```python
from build123d import *

# Parameters (mm, degrees)
F1_DEPTH  = 6
F3_DEPTH  = 130
F5_DEPTH  = 130
F7_DEPTH  = 130
F9_DEPTH  = 6
F10_R     = 41
F11_DEPTH = 309.88


with BuildPart() as f1:
    # F0 (on Front) → F1 (new body)
    with BuildSketch(Plane.XZ):
        Polygon((-110, 0), (0, 0), (110, 0), (0, 600), align=None)
    extrude(amount=F1_DEPTH)

    # F2 (on face) → F3 (join)
    with BuildSketch(Plane(origin=(0, 0, 0), x_dir=(-1, 0, 0), z_dir=(0, 1, 0))):
        Polygon((110, 0), (106.467944, 19.265758), (0, 600), (-3.05, 583.363636), (0, 566.727273), (88.482445, 84.095757), (103.9, 0), align=None)
    extrude(amount=F3_DEPTH)

    # F4 (on face) → F5 (join)
    with BuildSketch(Plane(origin=(0, 0, 0), x_dir=(-1, 0, 0), z_dir=(0, 1, 0))):
        Polygon((0, 566.727273), (-3.05, 583.363636), (-110, 0), (-103.9, 0), (-101.40299, 13.620052), align=None)
    extrude(amount=F5_DEPTH)

    # F6 (on face) → F7 (join)
    with BuildSketch(Plane(origin=(0, 0, 0), x_dir=(-1, 0, 0), z_dir=(0, 1, 0))):
        Polygon((-102.8, 6), (-103.9, 0), (103.9, 0), (102.8, 6), (94.243981, 6), (-89.78457, 6), align=None)
    extrude(amount=F7_DEPTH)

    # F8 (on face) → F9 (join)
    with BuildSketch(Plane(origin=(0, 130, 0), x_dir=(-1, 0, 0), z_dir=(0, 1, 0))):
        Polygon((110, 0), (0, 600), (-110, 0), align=None)
    extrude(amount=F9_DEPTH)

    # F10 (on face) → F11 (cut)
    with BuildSketch(Plane.XZ.offset(6)):
        with Locations((48.797943, 51.662218)):
            Circle(F10_R)
        with Locations((-51.237836, 50.848916)):
            Circle(F10_R)
        with Locations((-0.8133, 127.299026)):
            Circle(F10_R)
        with Locations((0, 217.074677)):
            Circle(F10_R)
        with Locations((0, 306.537598)):
            Circle(F10_R)
    extrude(amount=-F11_DEPTH, mode=Mode.SUBTRACT)


solid = f1.part
```
Input: part model. Units: mm. Frame: model coordinates. A direction names the side the tool comes from. Give positions to 0.01 mm unless a question says otherwise; leave off trailing zeros. Loops run counter-clockwise (first coordinate to the right, second up) from the corner with the lowest first, then second, coordinate; pieces in that order, holes last. Notation, with made-up numbers: (-4.5, 85.25) -> (13.5, 85.25) arc R21 cw to (13.5, 103.25) -> close; hole circle Ø5 at (31.5, -2). An arc over 180 degrees is marked (long way). Use a Markdown table: item, result.
Q1. Pull-direction query (Y, two-part tool) for faces 1 (the cylindrical face through (18.919, 132.958, 270.164)), 2 (the flat face through (16, -6, 257)), 3 (the flat face through (15, 0, 267)), 4 (the flat face through (17, 136, 257)); classes: pulls with the +Y half, pulls with the -Y half, needs draft (parallel to the pull), parting line crosses it, or undercut.
Entries:
| item | result |
|---|---|
| face 1 | needs draft |
| face 2 | pulls with the -Y half |
| face 3 | undercut |
| face 4 | pulls with the +Y half |
Q2. First-contact query: P1, Ø1, axis at y = 62, z = 442.5, coming from the -X side; P2, Ø10, axis at y = 41.5, z = 71.5, coming from the +X side; P3, Ø10, axis at y = 108.5, z = 471, coming from the -X side. Flat tips, straight axial feed; report the tip coordinate or a pass-through.
Entries:
| item | result |
|---|---|
| P1 | stops at x = -28.97 |
| P2 | stops at x = 97.81 |
| P3 | stops at x = -24.57 |
Q3. Section query A-A, the plane z = 438. Return the cut outline in (x, y), plus the area to 3 significant figures.
Entries:
| item | result |
|---|---|
| outline | (-29.7, -6) -> (29.7, -6) -> (29.7, 136) -> (-29.7, 136) -> close; hole (-23.6, 0) -> (23.6, 0) -> (23.6, 130) -> (-23.6, 130) -> close |
| area | 2,300 mm² |
Q4. Section query C-C, the plane x = 60. Return the cut outline in (y, z), plus the area to 3 significant figures.
Entries:
| item | result |
|---|---|
| outline | (-6, 0) -> (136, 0) -> (136, 12.22) -> (130, 12.22) -> (130, 6) -> (0, 6) -> (0, 12.22) -> (-6, 12.22) -> close; (-6, 91.1) -> (0, 91.1) -> (0, 239.45) -> (130, 239.45) -> (130, 91.1) -> (136, 91.1) -> (136, 272.73) -> (-6, 272.73) -> close |
| area | 7,430 mm² |
Q5. Section query D-D, the plane x = 17.5. State how many separate pieces and enclosed holes the cut face has, plus the area to 3 significant figures.
Entries:
| item | result |
|---|---|
| separate pieces | 8 |
| enclosed holes | 0 |
| area | 7,860 mm² |
Q6. Section query B-B, the plane y = 57. Return the cut outline in (x, z).
Entries:
| item | result |
|---|---|
| outline | (-110, 0) -> (110, 0) -> (0, 600) -> close; hole (-102.8, 6) -> (102.8, 6) -> (0, 566.73) -> close |
Q7. Ray query, probe 1 along Y at (x, z) = (-9.5, 507); probe 2 along X at (y, z) = (54.5, 103.5) (3 decimals); probe 3 along X at (y, z) = (31, 92). Return the intervals inside material, ascending. Write a range as from..to.
Entries:
| item | result |
|---|---|
| probe 1 | y = -6..0, 130..136 |
| probe 2 | x = -91.025..-84.925, 84.925..91.025 |
| probe 3 | x = -93.13..-87.03, 87.03..93.13 |
Q8. Access query for faces 5 (the flat face through (39, 130, 246)), 6 (the cylindrical face through (22.041, -3.042, 251.646)). Directions: +Z, -Z, +X, -X, +Y, -Y. A direction counts if a zero-diameter tool reaches every point of the face in a straight line with its end or side. Return the directions, or none.
Entries:
| item | result |
|---|---|
| face 5 | none |
| face 6 | +Y, -Y |
